```python
from build123d import *

# Parameters (mm, degrees)
F0_W     = 304.8
F0_H     = 50.8
F1_DEPTH = 6.35
F2_W     = 3.175
F2_H     = 50.8
F3_DEPTH = 3.175


with BuildPart() as f1:
    # F0 (on Right) → F1 (new body)
    with BuildSketch(Plane.YZ):
        with Locations((21.336002, -28.165208)):
            Rectangle(F0_W, F0_H)
    extrude(amount=F1_DEPTH)

    # F2 (on face) → F3 (cut)
    with BuildSketch(Plane.YZ.offset(6.35)):
        with Locations((-69.151498, -28.165208)):
            Rectangle(F2_W, F2_H)
        with Locations((-8.826498, -28.165208)):
            Rectangle(F2_W, F2_H)
        with Locations((51.498502, -28.165208)):
            Rectangle(F2_W, F2_H)
        with Locations((111.823502, -28.165208)):
            Rectangle(F2_W, F2_H)
    extrude(amount=-F3_DEPTH, mode=Mode.SUBTRACT)


solid = f1.part
```
Can you work these out from the model? Positions are in its coordinate system, mm. Round coordinates to 2 decimals unless told otherwise and drop trailing zeros. Order: outer loops, then holes, each group sorted by start corner. A loop starts at its lowest first (then second) coordinate and runs counter-clockwise, first axis right, second up.
(1) If I drill on L1, parallel to Y at x = 4, z = -14, over which ranges is the centre line in solid material (lowest first)?
Results are:
L1: y = -131.06 to -70.74, -67.56 to -10.41, -7.24 to 49.91, 53.09 to 110.24, 113.41 to 173.74
(2) I'm going to push flat-ended pins straight in: pin 1 (3.5 mm diameter, centred on y = -70, z = -33.5, fed in from +X); pin 2 (1.6 mm diameter, centred on y = -9, z = -26, fed in from +X) (3 decimals). Where does each tip first touch, or does it pass through?
Results are:
pin 1: stops at x = 6.35
pin 2: stops at x = 3.175
(3) If we section it at A-A (z = -46.5): Please give me the cut outline in (x, y) (3 decimals), plus the area to 3 significant figures.
Results are:
outline: (0, -131.064) - (6.35, -131.064) - (6.35, -70.739) - (3.175, -70.739) - (3.175, -67.564) - (6.35, -67.564) - (6.35, -10.414) - (3.175, -10.414) - (3.175, -7.239) - (6.35, -7.239) - (6.35, 49.911) - (3.175, 49.911) - (3.175, 53.086) - (6.35, 53.086) - (6.35, 110.236) - (3.175, 110.236) - (3.175, 113.411) - (6.35, 113.411) - (6.35, 173.736) - (0, 173.736) - close
area: 1,900 mm2
